Here's how the part is built. I have some questions about the finished solid (model axes, mm). A direction names the side the tool comes from. Give positions to 0.01 mm unless a question says otherwise; leave off trailing zeros. Return JSON: item names as keys, results as strings. Group by question number.
(1) On a 3-axis mill with a long thin cutter (end or side, diameter ignored), from which of +Z, -Z, +X, -X, +Y, -Y can I reach the whole of each face in a straight line? I mean faces 1 (the flat face through (15, 10.16, -23)), 2 (the flat face through (-35.716, 8, -23)). Say none if no direction works.
(2) For P1, Ø1.4, axis at x = 14, z = -23.5, coming from the -Y side, with a flat end and sliding along its axis, tell me the tip position at first contact or that it passes through.
(3) If we mould it in two halves opening along Z, with no side actions, what happens to faces 3 (the flat face through (14, 8, -74.033)), 4 (the cylindrical face through (17.12, 5.01, -24.53)), 5 (the flat face through (14, 8, 27.567)), 6 (the flat face through (65.884, 8, -23))? For each: released by +Z, released by -Z, zero draft, split by the parting line, or undercut.
(4) I need wall thicknesses on probe 1 along Z at (x, y) = (14, 8.5). Which ranges of the line are inside material? Lowest first, please. Write a range as [from, to].
```python
from build123d import *

# Parameters (mm, degrees)
SKETCH1_W           = 101.6
SKETCH1_H           = 101.6
BOSS_EXTRUDE1_DEPTH = 15.24
SKETCH2_R           = 2.413
CUT_EXTRUDE1_DEPTH  = 10.16


with BuildPart() as part:
    # Sketch1 → Boss-Extrude1 (new body)
    with BuildSketch(Plane(origin=(0, 0, 0), x_dir=(1, 0, 0), z_dir=(0, 1, 0))):
        with Locations((15.083959044, 23.232764505)):
            Rectangle(SKETCH1_W, SKETCH1_H)
    extrude(amount=BOSS_EXTRUDE1_DEPTH)

    # Sketch2 → Cut-Extrude1 (cut)
    with BuildSketch(Plane.XZ):
        with Locations(Location((15.083959044, -23.232764505, 0), (0, 0, 270))):
            Circle(SKETCH2_R)
    extrude(amount=-CUT_EXTRUDE1_DEPTH, mode=Mode.SUBTRACT)


solid = part.part
```
Values:
{
 "1": {"face 1": "-Y", "face 2": "+Z, -Z, -X, +Y, -Y"},
 "2": {"P1": "y = 10.16"},
 "3": {"face 3": "released by -Z", "face 4": "undercut", "face 5": "released by +Z", "face 6": "zero draft"},
 "4": {"probe 1": "[-74.03, -25.39], [-21.08, 27.57]"}
}
